Build history of the part. All positions in model axes, mm. A direction names the side the tool comes from. Give positions to 0.01 mm unless a question says otherwise; leave off trailing zeros. Write each loop counter-clockwise with the first axis right and the second up, starting at its lowest first coordinate (ties: lowest second). Pieces come first, ordered by that corner, then holes.
Autodesk Inventor part; units mm, degrees
ref_plane "Work Plane1" through (0, 34.29, 0) normal (0, 1, 0) x (1, 0, 0)
ref_plane "YZ Plane" through (0, 0, 0) normal (1, 0, 0) x (0, 1, 0)
ref_plane "XZ Plane" through (0, 0, 0) normal (0, 1, 0) x (-1, 0, 0)
sketch "Sketch2" plane through (0, 0, 0) normal (0, 1, 0) x (-1, 0, 0)
  line L0 (-27.178, 13.97) -> (27.178, 13.97)
  line L1 (27.178, 13.97) -> (27.178, -13.97)
  line L2 (27.178, -13.97) -> (-27.178, -13.97)
  line L3 (-27.178, -13.97) -> (-27.178, 13.97)
  line L4 (-27.178, 13.97) -> (27.178, -13.97) construction
  point P0 (0, 0)
  point P1 (0, 0)
  dimension "d0" = 54.356
  dimension "d1" = 27.94
extrude "Extrusion1" add sketch "Sketch2" along normal blind 12.954
sketch "Sketch3" plane through (-27.178, 0, 13.97) normal (0, 0, 1) x (1, 0, 0)
  line L0 (54.356, 12.954) -> (0, 12.954)
  line L1 (0, 0) -> (0, 12.954)
  line L2 (54.356, 0) -> (0, 0)
  line L3 (4.826, 11.684) -> (5.588, 11.684)
  line L4 (5.588, 11.684) -> (5.588, 3.81)
  line L5 (5.588, 3.81) -> (4.826, 3.81)
  line L6 (4.826, 3.81) -> (4.826, 11.684)
  line L7 (14.986, 11.684) -> (15.748, 11.684)
  line L8 (15.748, 11.684) -> (15.748, 3.81)
  line L9 (15.748, 3.81) -> (14.986, 3.81)
  line L10 (14.986, 3.81) -> (14.986, 11.684)
  line L11 (25.146, 11.684) -> (25.908, 11.684)
  line L12 (25.908, 11.684) -> (25.908, 3.81)
  line L13 (25.908, 3.81) -> (25.146, 3.81)
  line L14 (25.146, 3.81) -> (25.146, 11.684)
  line L15 (35.306, 11.684) -> (36.068, 11.684)
  line L16 (36.068, 11.684) -> (36.068, 3.81)
  line L17 (36.068, 3.81) -> (35.306, 3.81)
  line L18 (35.306, 3.81) -> (35.306, 11.684)
  line L19 (45.466, 11.684) -> (46.228, 11.684)
  line L20 (46.228, 11.684) -> (46.228, 3.81)
  line L21 (46.228, 3.81) -> (45.466, 3.81)
  line L22 (45.466, 3.81) -> (45.466, 11.684)
  point P0 (27.178, 0)
  dimension "d4" = 0.762
  dimension "d5" = 7.874
  dimension "d6" = 1.27
  dimension "d7" = 4.826
  dimension "d10" = 10.16
extrude "Extrusion2" add sketch "Sketch3" along normal blind 9.398
sketch "Sketch4" plane through (-22.352, 3.81, 13.97) normal (-1, 0, 0) x (0, 0, 1)
  line L0 (0, 0) -> (0, 7.874)
  line L1 (1.524, 7.874) -> (9.398, 7.874)
  line L2 (9.398, 7.874) -> (9.398, 7.112)
  line L3 (9.398, 7.112) -> (1.524, 7.112)
  line L4 (1.524, 7.112) -> (1.524, 7.874)
  line L5 (9.398, 0) -> (1.524, 0)
  line L6 (1.524, 0) -> (1.524, 0.762)
  line L7 (1.524, 0.762) -> (9.398, 0.762)
  line L8 (9.398, 0.762) -> (9.398, 0)
  circle A0 centre (5.461, 3.937) radius 0.762
  line L9 (9.398, 7.112) -> (1.524, 0.762) construction
  point P0 (-13.97, -3.81)
  dimension "d17" = 6.35
  dimension "d18" = 1.524
  dimension "d19" = 1.524
extrude "Extrusion3" cut sketch "Sketch4" against normal up to surface (41.402 mm away)
mirror "Mirror1" about plane through (0, 0, 0) normal (0, 0, 1) of "Extrusion2", "Extrusion3"
sketch "Sketch5" plane through (0, 12.954, 0) normal (0, 1, 0) x (1, 0, 0)
  line L0 (-27.178, -13.97) -> (-27.178, 13.97)
  line L1 (27.178, -13.97) -> (-27.178, -13.97)
  line L2 (-27.178, 13.97) -> (27.178, 13.97)
  line L3 (27.178, 13.97) -> (27.178, -13.97)
  line L4 (27.178, -13.97) -> (-27.178, -13.97)
  line L5 (-27.178, -13.97) -> (-27.178, 13.97)
  point P0 (0, 0)
ref_plane "Work Plane1" through (0, 34.29, 0) normal (0, 1, 0) x (1, 0, 0)
sketch "Sketch6" plane through (0, 34.29, 0) normal (0, 1, 0) x (1, 0, 0)
  line L0 (-27.178, 12.7) -> (27.178, 12.7)
  line L1 (27.178, 12.7) -> (27.178, -12.7)
  line L2 (27.178, -12.7) -> (-27.178, -12.7)
  line L3 (-27.178, -12.7) -> (-27.178, 12.7)
  line L4 (27.178, 12.7) -> (-27.178, -12.7) construction
  point P0 (0, 0)
  point P1 (0, 0)
  point P2 (-27.178, 13.97)
  dimension "d23" = 25.4
loft "Loft1" add profiles "Sketch5", "Sketch6"
properties part number "FuseBlock"
(1) Saw through at D-D, the plane y = 31.5. List the corners of the cut face in (x, z).
(2) Mould opens along Y. For faces 4 (the face through (-21.98, 8.49, -19.27)), 5 (the face through (-22.352, 8, -18)), 6 (the face through (0.38, 23.771, -13.326)), 7 (the face through (18.66, 8.49, -19.27)) say: +Y half, -Y half, draft (parallel to the pull), parting line (faces both ways), or undercut.
(3) Saw through at A-A, the plane z = 17. List the corners of the cut face in (x, y).
(4) Drop flat-ended pins along their axis: pin 1 (1.4 mm diameter, centred on y = 7.747, z = -19.431, fed in from -X); pin 2 (0.8 mm diameter, centred on x = -22, z = 18.5, fed in from +Y); pin 3 (4 mm diameter, centred on y = 6.5, z = -18, fed in from +X); pin 4 (6 mm diameter, centred on x = -12.5, y = 23, fed in from -Z). Give the stop position or say it passes through.
(5) 3-axis set-ups, long thin cutter, end or side, ignore diameter. For faces 1 (the face through (-21.59, 8, 18)), 2 (the face through (19.05, 8, -18)), 3 (the face through (-12.192, 8, -18)): which of +Z, -Z, +X, -X, +Y, -Y reach the whole face in a straight line?
(6) Saw through at B-B, the plane x = -9. List the corners of the cut face in (y, z), plus the area to 3 significant figures.
(7) Probe line 1 (X direction, y = 5, z = 16); line 2 (Z direction, x = 24, y = 7); line 3 (Z direction, x = -0.5, y = 29). List the from-to ranges inside material, lowest first.
(8) Saw through at C-C, the plane y = 3. List the corners of the cut face in (x, z), plus the area to 3 significant figures.
Computed values:
1. outline: (-27.18, -12.87) - (27.18, -12.87) - (27.18, 12.87) - (-27.18, 12.87) - close
2. face 4: undercut
2. face 5: draft
2. face 6: +Y half
2. face 7: undercut
3. outline: (-22.35, 4.57) - (-21.59, 4.57) - (-21.59, 10.92) - (-22.35, 10.92) - close; (-12.19, 4.57) - (-11.43, 4.57) - (-11.43, 10.92) - (-12.19, 10.92) - close; (-2.03, 4.57) - (-1.27, 4.57) - (-1.27, 10.92) - (-2.03, 10.92) - close; (8.13, 4.57) - (8.89, 4.57) - (8.89, 10.92) - (8.13, 10.92) - close; (18.29, 4.57) - (19.05, 4.57) - (19.05, 10.92) - (18.29, 10.92) - close
4. pin 1: passes through
4. pin 2: stops at y = 10.92
4. pin 3: stops at x = 19.05
4. pin 4: stops at z = -13.55
5. face 1: +Z, +Y, -Y
5. face 2: -Z, +X, +Y, -Y
5. face 3: -Z, +Y, -Y
6. outline: (0, -13.97) - (12.95, -13.97) - (34.29, -12.7) - (34.29, 12.7) - (12.95, 13.97) - (0, 13.97) - close
6. area: 931 mm2
7. line 1: x = -22.35 to -21.59, -12.19 to -11.43, -2.03 to -1.27, 8.13 to 8.89, 18.29 to 19.05
7. line 2: z = -13.97 to 13.97
7. line 3: z = -13.01 to 13.01
8. outline: (-27.18, -13.97) - (27.18, -13.97) - (27.18, 13.97) - (-27.18, 13.97) - close
8. area: 1,520 mm2
